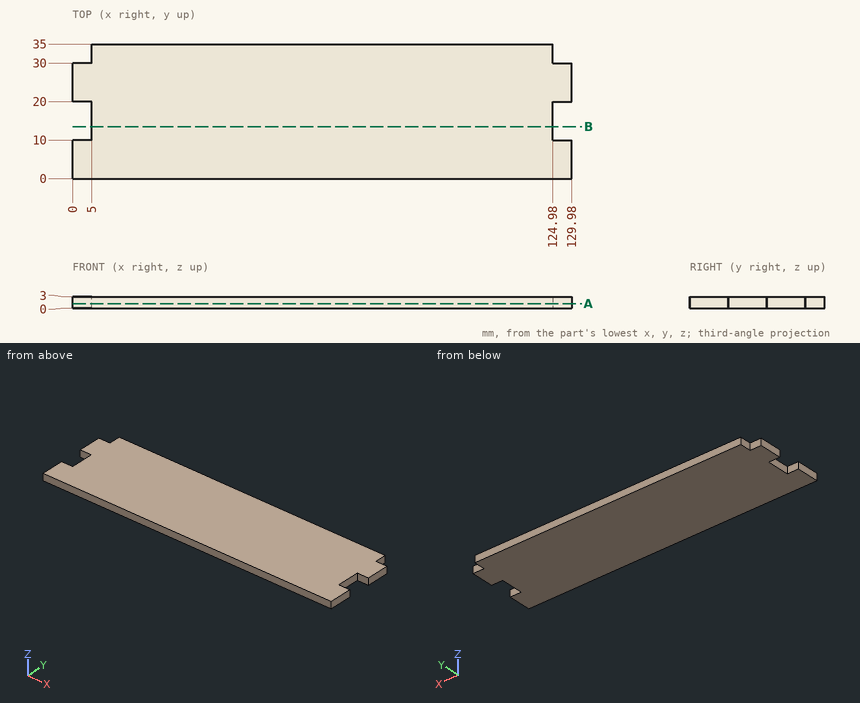
Could you check a few things on this drawing? It's one solid part, dimensions in mm from its lowest x, y, z. Coordinates: 2 decimals unless noted, no trailing zeros. Order: outer loops, then holes, each group sorted by start corner. A loop starts at its lowest first (then second) coordinate and runs counter-clockwise, first axis right, second up. Notation, with made-up numbers: M 68,60.25 L 75,60.25 A3 ccw 75,64.25 Z; hole C -12.75,7.5 d10. An arc over 180 degrees is marked long. Answer as a JSON object with one key per item and string values. Group by question number.
(1) I need wall thicknesses on probe 1 along X at (y, z) = (17.5, 1.7). Which ranges of the line are inside material? Lowest first, please.
(2) For pin 1 (1.5 mm diameter, centred on x = 2.5, z = 1, fed in from +Y); pin 2 (1.5 mm diameter, centred on y = 16, z = 2, fed in from +X); pin 3 (1.5 mm diameter, centred on y = 32, z = 1, fed in from -X), each with a flat end and sliding along its axis, tell me the tip position at first contact or that it passes through.
(3) Suppose I cut it at B-B, the plane y = 13.5. Please give me the cut outline in (x, z).
(4) Suppose I cut it at A-A, the plane z = 1.15. Please give me the cut outline in (x, y).
Values found:
{
 "1": {"probe 1": "x = 5 to 124.98"},
 "2": {"pin 1": "stops at y = 30", "pin 2": "stops at x = 124.98", "pin 3": "stops at x = 5"},
 "3": {"outline": "M 5,0 L 124.98,0 L 124.98,3 L 5,3 Z"},
 "4": {"outline": "M 0,0 L 129.98,0 L 129.98,10 L 124.98,10 L 124.98,20 L 129.98,20 L 129.98,30 L 124.98,30 L 124.98,35 L 5,35 L 5,30 L 0,30 L 0,20 L 5,20 L 5,10 L 0,10 Z"}
}
